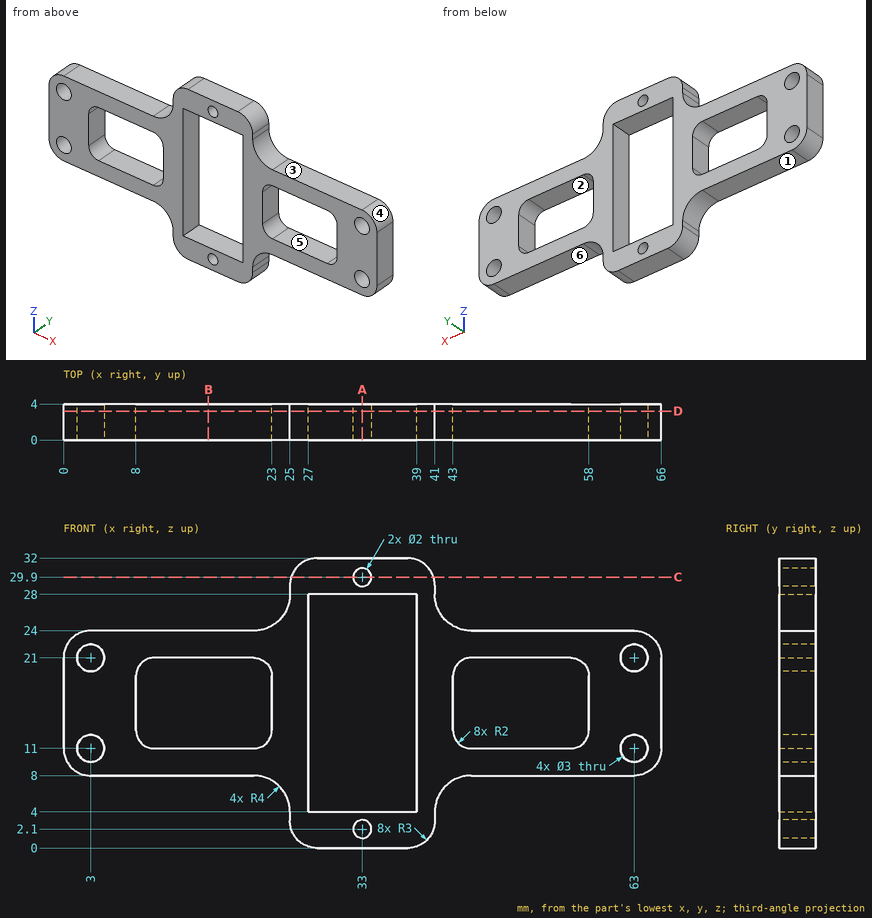
Job drawing, mm, ordinate dimensions from the low corner. One solid piece. A direction names the side the tool comes from. Give positions to 0.01 mm unless a question says otherwise; leave off trailing zeros. Write each loop counter-clockwise with the first axis right and the second up, starting at its lowest first coordinate (ties: lowest second). Pieces come first, ordered by that corner, then holes. Notation, with made-up numbers: M 4.5,-6.5 L 32.5,-6.5 A6 cw 32.5,2.5 Z; hole C 62,-12 d10. An arc over 180 degrees is marked long. One line per item, written item: value. Start each with the question number.
Q1. Saw through at D-D, the plane y = 3.2. State how many separate pieces and enclosed holes the cut face has, plus the area to 3 significant figures.
Q2. Two-plate mould, pull along X, no slides. Class the marked faces 4, 5 and 6: +X half, -X half, draft (parallel to the pull), parting line (faces both ways), or undercut.
Q3. 3-axis set-ups, long thin cutter, end or side, ignore diameter. For the marked faces 1, 2 and 3: which of +Z, -Z, +X, -X, +Y, -Y reach the whole face in a straight line?
Q4. Drop flat-ended pins along their axis: pin 1 Ø0.5 at (y, z) = (3, 28.5) entering from -X; pin 2 Ø1.2 at (x, y) = (15, 1.5) entering from -Z. Give the stop position or say it passes through.
Q5. Saw through at B-B, the plane x = 16. Write the cut outline in (y, z), plus the area to 3 significant figures.
Q6. Probe probe 1 along X at (y, z) = (2.9, 13); probe 2 along Z at (x, y) = (33, 2.45); probe 3 along Z at (x, y) = (63, 2.6). List the from-to ranges inside material, lowest first. Write a range as [from, to].
Q7. Saw through at A-A, the plane x = 33. Write the cut outline in (y, z).
Q8. Saw through at C-C, the plane z = 29.9. Write the cut outline in (x, y), plus the area to 3 significant figures.
Output values:
1. separate pieces: 1
1. enclosed holes: 9
1. area: 695 mm²
2. face 4: +X half
2. face 5: undercut
2. face 6: draft
3. face 1: -Z, -X, +Y, -Y
3. face 2: +Y, -Y
3. face 3: +Z, +X, +Y, -Y
4. pin 1: stops at x = 25
4. pin 2: stops at z = 8
5. outline: M 0,8 L 4,8 L 4,11 L 0,11 Z; M 0,21 L 4,21 L 4,24 L 0,24 Z
5. area: 24.0 mm²
6. probe 1: x = [0, 8], [23, 27], [39, 43], [58, 66]
6. probe 2: z = [0, 1.1], [3.1, 4], [28, 28.9], [30.9, 32]
6. probe 3: z = [8, 9.5], [12.5, 19.5], [22.5, 24]
7. outline: M 0,0 L 4,0 L 4,1.1 L 0,1.1 Z; M 0,3.1 L 4,3.1 L 4,4 L 0,4 Z; M 0,28 L 4,28 L 4,28.9 L 0,28.9 Z; M 0,30.9 L 4,30.9 L 4,32 L 0,32 Z
8. outline: M 25.14,0 L 32,0 L 32,4 L 25.14,4 Z; M 34,0 L 40.86,0 L 40.86,4 L 34,4 Z
8. area: 54.9 mm²
